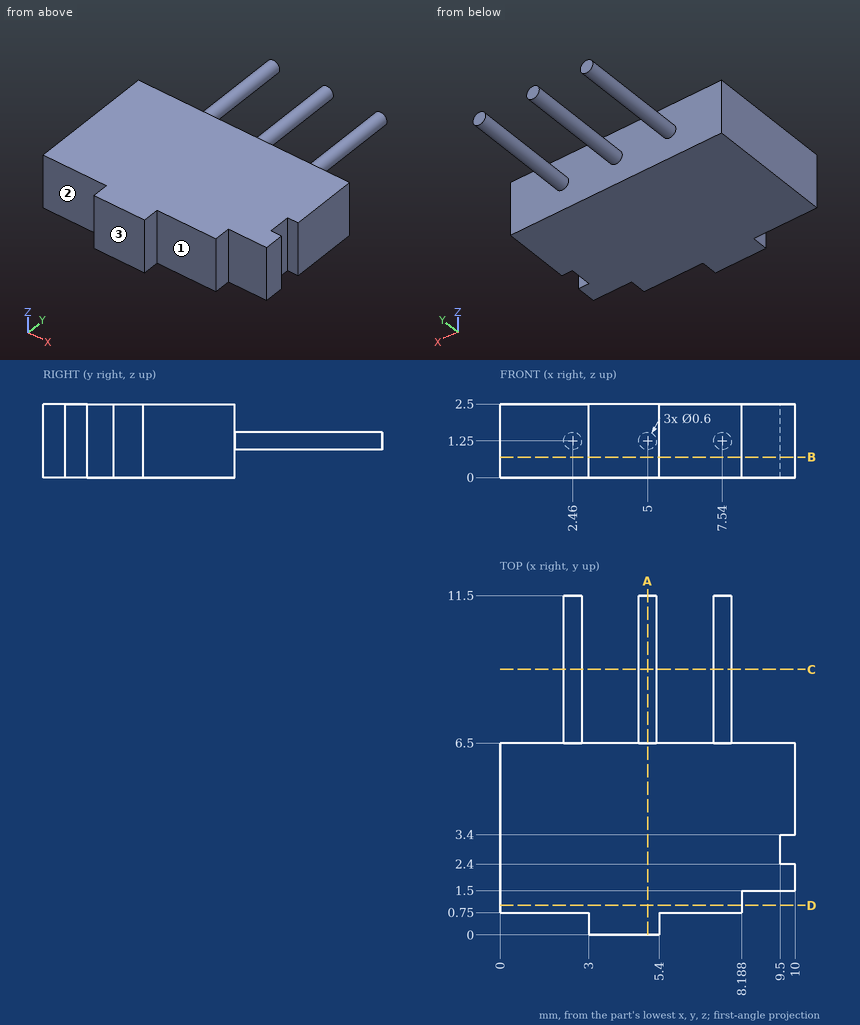
Input: dimensioned drawing with shaded views. Units: mm. Origin: part minimum x, y, z. A direction names the side the tool comes from. Give positions to 0.01 mm unless a question says otherwise; leave off trailing zeros. Loops run counter-clockwise (first coordinate to the right, second up) from the corner with the lowest first, then second, coordinate; pieces in that order, holes last. Notation, with made-up numbers: (76, 66.5) - (83, 66.5) arc R10 ccw to (83, 80.5) - close; hole circle Ø2 at (38.25, 41). An arc over 180 degrees is marked (long way). Answer as CSV lines item,"result". Start each with the question number.
(1) Section query B-B (z = 0.7). Output: boundary loops of the cut face in (x, y).
(2) Ray query, line 1 along Y through (x, z) = (7, 2.1); line 2 along X through (y, z) = (1, 0.15); line 3 along Y through (x, z) = (4.25, 0.2). Return the intervals inside material, ascending. Write a range as [from, to].
(3) Section query A-A (x = 5). Output: boundary loops of the cut face in (y, z).
(4) Section query D-D (y = 1). Output: boundary loops of the cut face in (x, z), and give its area (3 significant figures).
(5) Reachability of the marked faces 1, 2 and 3 from +Z, -Z, +X, -X, +Y, -Y: full face, straight path, thin tool, end or side. Return the list, or none.
(6) Pin query (flat end, axial travel): P1, Ø1.5, axis at x = 3.5, z = 0.5, coming from the +Y side; P2, Ø1.5, axis at x = 7.5, z = 0.5, coming from the -Y side; P3, Ø0.6, axis at y = 1, z = 1, coming from the +X side. Return the tip coordinate at first contact, or that it passes through.
(7) Section query C-C (y = 9). Output: boundary loops of the cut face in (x, z).
Worked answers:
1,outline,"(0, 0.75) - (3, 0.75) - (3, 0) - (5.4, 0) - (5.4, 0.75) - (8.19, 0.75) - (8.19, 1.5) - (10, 1.5) - (10, 2.4) - (9.5, 2.4) - (9.5, 3.4) - (10, 3.4) - (10, 6.5) - (0, 6.5) - close"
2,line 1,"y = [0.75, 6.5]"
2,line 2,"x = [0, 8.19]"
2,line 3,"y = [0, 6.5]"
3,outline,"(0, 0) - (6.5, 0) - (6.5, 0.95) - (11.5, 0.95) - (11.5, 1.55) - (6.5, 1.55) - (6.5, 2.5) - (0, 2.5) - close"
4,outline,"(0, 0) - (8.19, 0) - (8.19, 2.5) - (0, 2.5) - close"
4,area,"20.5 mm^2"
5,face 1,"+Z, -Z, +X, -Y"
5,face 2,"+Z, -Z, -X, -Y"
5,face 3,"+Z, -Z, +X, -X, -Y"
6,P1,"stops at y = 6.5"
6,P2,"stops at y = 0.75"
6,P3,"stops at x = 8.19"
7,outline,"circle Ø0.6 at (2.46, 1.25); circle Ø0.6 at (5, 1.25); circle Ø0.6 at (7.54, 1.25)"
